Build history of the part. All positions in model axes, mm. Coordinates: 2 decimals unless noted, no trailing zeros. Loops run counter-clockwise (first coordinate to the right, second up) from the corner with the lowest first, then second, coordinate; pieces in that order, holes last.
Item 1: Flat gauge pins, fed straight in: pin 1 (5.5 mm diameter, centred on x = -27.43, z = 30.27, fed in from +Y); pin 2 (8 mm diameter, centred on x = 4, z = -24.5, fed in from +Y). Where does each tip first touch, or does it go through?
Item 2: Cut at C-C (z = -30.27). List the corners of the cut face in (x, y).
Item 3: Cut at D-D (y = 1.15). Count the separate pieces of the cut face and the enclosed holes in it, and give its area (3 significant figures).
Item 4: Cut at A-A (z = 0). List the corners of the cut face in (x, y), and give its area (3 significant figures).
Item 5: Cut at B-B (x = 0). List the corners of the cut face in (y, z).
Item 6: Drill centre lines: line 1 along X through (y, z) = (0.7, -30.27); line 2 along Z through (x, y) = (26.5, 1.2); line 3 along X through (y, z) = (1.9, -26). Where is each one in solid material? Low to high.
from build123d import *

# Parameters (mm, degrees)
SKETCH_1_W          = 62
SKETCH_1_H          = 67
SKETCH_1_R          = 2
EXTRUDE_1_DEPTH     = 2
SKETCH_4_R          = 29
CUT_EXTRUDE_2_DEPTH = 2
SKETCH_5_R          = 1.75
CUT_EXTRUDE_3_DEPTH = 2


with BuildPart() as part:
    # Эскиз1 → Бобышка-Вытянуть1 (new body)
    with BuildSketch(Plane(origin=(0, 0, 0), x_dir=(1, 0, 0), z_dir=(0, 1, 0))):
        Rectangle(SKETCH_1_W, SKETCH_1_H)
        with Locations(Location((25, 25, 0), (0, 0, 270))):
            Circle(SKETCH_1_R, mode=Mode.SUBTRACT)
        with Locations(Location((-25, 25, 0), (0, 0, 270))):
            Circle(SKETCH_1_R, mode=Mode.SUBTRACT)
        with Locations(Location((25, -25, 0), (0, 0, 270))):
            Circle(SKETCH_1_R, mode=Mode.SUBTRACT)
        with Locations(Location((-25, -25, 0), (0, 0, 270))):
            Circle(SKETCH_1_R, mode=Mode.SUBTRACT)
    extrude(amount=EXTRUDE_1_DEPTH)

    # Эскиз4 → Вырез-Вытянуть2 (cut)
    with BuildSketch(Plane.XZ):
        with Locations(Location((0, 0, 0), (0, 0, 270))):
            Circle(SKETCH_4_R)
    extrude(amount=-CUT_EXTRUDE_2_DEPTH, mode=Mode.SUBTRACT)

    # Эскиз5 → Вырез-Вытянуть3 (cut)
    with BuildSketch(Plane.XZ):
        with Locations(Location((-27.43, 30.27, 0), (0, 0, 270))):
            Circle(SKETCH_5_R)
        with Locations(Location((-27.43, -30.27, 0), (0, 0, 90))):
            Circle(SKETCH_5_R)
        with Locations(Location((27.43, -30.27, 0), (0, 0, 270))):
            Circle(SKETCH_5_R)
        with Locations(Location((27.43, 30.27, 0), (0, 0, 90))):
            Circle(SKETCH_5_R)
    extrude(amount=-CUT_EXTRUDE_3_DEPTH, mode=Mode.SUBTRACT)


solid = part.part
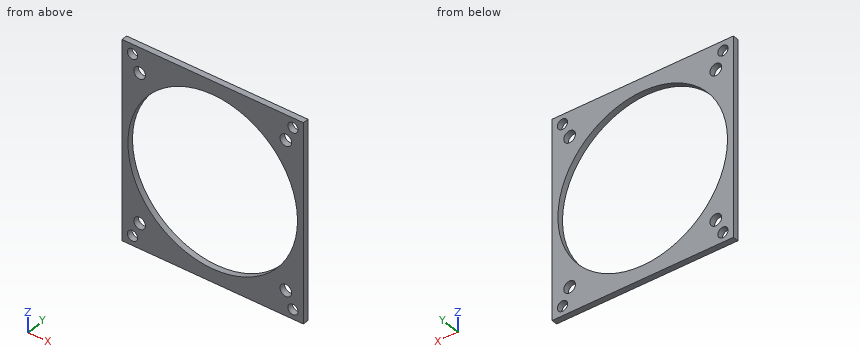
Filled sheet:
1. pin 1: stops at y = 2
1. pin 2: passes through
2. outline: (-31, 0) - (-29.18, 0) - (-29.18, 2) - (-31, 2) - close; (-25.68, 0) - (25.68, 0) - (25.68, 2) - (-25.68, 2) - close; (29.18, 0) - (31, 0) - (31, 2) - (29.18, 2) - close
3. separate pieces: 1
3. enclosed holes: 9
3. area: 1,420 mm2
4. outline: (-31, 0) - (-29, 0) - (-29, 2) - (-31, 2) - close; (29, 0) - (31, 0) - (31, 2) - (29, 2) - close
4. area: 8.00 mm2
5. outline: (0, -33.5) - (2, -33.5) - (2, -29) - (0, -29) - close; (0, 29) - (2, 29) - (2, 33.5) - (0, 33.5) - close
6. line 1: x = -31 to -29.18, -25.68 to 25.68, 29.18 to 31
6. line 2: z = -33.5 to -31.75, -28.79 to -26.32, -23.68 to -11.78, 11.78 to 23.68, 26.32 to 28.79, 31.75 to 33.5
6. line 3: x = -31 to -26.73, -23.27 to -12.85, 12.85 to 23.27, 26.73 to 31
